Read the model definition and answer for the solid it produces. Units are mm, in the model's axes. A direction names the side the tool comes from. Give positions to 0.01 mm unless a question says otherwise; leave off trailing zeros. Order: outer loops, then holes, each group sorted by start corner. A loop starts at its lowest first (then second) coordinate and runs counter-clockwise, first axis right, second up. Notation, with made-up numbers: (15.5, -2) - (55.5, -2) arc R15 cw to (55.5, 27) - close; hole circle Ø11 at (-39.75, 12). An arc over 180 degrees is marked (long way). Return JSON: item names as keys, results as strings.
Autodesk Inventor part; units mm, degrees
ref_plane "YZ Plane" through (0, 0, 0) normal (1, 0, 0) x (0, 1, 0)
ref_plane "XZ Plane" through (0, 0, 0) normal (0, 1, 0) x (-1, 0, 0)
ref_plane "XY Plane" through (0, 0, 0) normal (0, 0, 1) x (1, 0, 0)
sketch "Sketch1" plane through (0, 0, 0) normal (0, 1, 0) x (-1, 0, 0)
  line L0 (-38.1, 0) -> (38.1, 0)
  line L1 (38.1, 0) -> (38.1, -25.4)
  line L2 (38.1, -25.4) -> (12.7, -25.4)
  line L3 (12.7, -25.4) -> (12.7, -88.9)
  line L4 (12.7, -88.9) -> (-12.7, -88.9)
  line L5 (-12.7, -88.9) -> (-12.7, -25.4)
  line L6 (-12.7, -25.4) -> (-38.1, -25.4)
  line L7 (-38.1, -25.4) -> (-38.1, 0)
  circle A0 centre (0, -12.7) radius 2.4892
  circle A1 centre (25.4, -12.7) radius 2.4892
  line L8 (0, 0) -> (0, -88.9) construction
  circle A2 centre (-25.4, -12.7) radius 2.4892
  circle A3 centre (0, -44.45) radius 2.4892
  circle A4 centre (0, -69.85) radius 2.4892
  point P0 (38.1, -12.7)
  point P1 (0, -44.45)
  dimension "d0" = 76.2
  dimension "d1" = 25.4
  dimension "d2" = 25.4
  dimension "d3" = 63.5
  dimension "d4" = 4.9784
  dimension "d5" = 25.4
  dimension "d6" = 31.75
  dimension "d7" = 25.4
extrude "Extrusion1" add sketch "Sketch1" along normal blind 6.35
fillet "Fillet1" radius 6.35 8 edges at (-38.1, 3.175, 0) (-38.1, 3.175, -25.4) (-12.7, 3.175, -25.4) (-12.7, 3.175, -88.9) (12.7, 3.175, -88.9) (12.7, 3.175, -25.4) (38.1, 3.175, -25.4) (38.1, 3.175, 0)
properties part number "STRU_020_DVBSBracket1" material "Aluminum 6061"
Q1. A cutting plane is placed at C-C (x = 25.4). Write down the section's boundary in (y, z).
Values:
{"outline": "(0, -25.4) - (6.35, -25.4) - (6.35, -15.19) - (0, -15.19) - close; (0, -10.21) - (6.35, -10.21) - (6.35, 0) - (0, 0) - close"}
Q2. Consider L1, parallel to Z at x = 0, y = 2.5; L2, parallel to X at y = 4, z = -13; L3, parallel to X at y = 6, z = -76.5. Determine where each line is inside the solid, lowest interval first.
Values:
{"L1": "z = -88.9 to -72.34, -67.36 to -46.94, -41.96 to -15.19, -10.21 to 0", "L2": "x = -38.1 to -27.87, -22.93 to -2.47, 2.47 to 22.93, 27.87 to 38.1", "L3": "x = -12.7 to 12.7"}
Q3. Given pin 1 (1.5 mm diameter, centred on y = 0.5, z = -65.5, fed in from -X); pin 2 (3 mm diameter, centred on y = 3, z = -69, fed in from +X); pin 3 (3 mm diameter, centred on x = 28, y = 2.5, fed in from -Z), each flat-ended and moving along its own axis, determine where each tip first touches the part or whether it passes through.
Values:
{"pin 1": "stops at x = -12.7", "pin 2": "stops at x = 12.7", "pin 3": "stops at z = -25.4"}
Q4. A cutting plane is placed at B-B (z = -69.85). Write down the section's boundary in (x, y), and give its area (3 significant figures).
Values:
{"outline": "(-12.7, 0) - (-2.49, 0) - (-2.49, 6.35) - (-12.7, 6.35) - close; (2.49, 0) - (12.7, 0) - (12.7, 6.35) - (2.49, 6.35) - close", "area": "130 mm²"}
Q5. For faces 1 (the flat face through (-12.7, 3, -57)), 2 (the flat face through (0, 3, 0)), 3 (the flat face through (25, 3, -25.4)), determine the directions among +Z, -Z, +X, -X, +Y, -Y from which every point of the face is accessible in a straight line to the end or side of a thin tool.
Values:
{"face 1": "-Z, -X, +Y, -Y", "face 2": "+Z, +X, -X, +Y, -Y", "face 3": "-Z, +X, +Y, -Y"}
Q6. Determine the mould class of faces 4 (the flat face through (-25, 3, -25.4)), 5 (the flat face through (12.7, 3, -58)), 6 (the cylindrical face through (-26.74, 3.13, -14.8)) for opening direction Z: released by +Z, released by -Z, zero draft, split by the parting line, or undercut.
Values:
{"face 4": "released by -Z", "face 5": "zero draft", "face 6": "undercut"}
Q7. A cutting plane is placed at A-A (x = 0). Write down the section's boundary in (y, z), and give its area (3 significant figures).
Values:
{"outline": "(0, -88.9) - (6.35, -88.9) - (6.35, -72.34) - (0, -72.34) - close; (0, -67.36) - (6.35, -67.36) - (6.35, -46.94) - (0, -46.94) - close; (0, -41.96) - (6.35, -41.96) - (6.35, -15.19) - (0, -15.19) - close; (0, -10.21) - (6.35, -10.21) - (6.35, 0) - (0, 0) - close", "area": "470 mm²"}
Q8. A cutting plane is placed at D-D (y = 1.75). Write down the section's boundary in (x, z).
Values:
{"outline": "(-38.1, -19.05) arc R6.35 ccw to (-31.75, -25.4) - (-19.05, -25.4) arc R6.35 cw to (-12.7, -31.75) - (-12.7, -82.55) arc R6.35 ccw to (-6.35, -88.9) - (6.35, -88.9) arc R6.35 ccw to (12.7, -82.55) - (12.7, -31.75) arc R6.35 cw to (19.05, -25.4) - (31.75, -25.4) arc R6.35 ccw to (38.1, -19.05) - (38.1, -6.35) arc R6.35 ccw to (31.75, 0) - (-31.75, 0) arc R6.35 ccw to (-38.1, -6.35) - close; hole circle Ø4.98 at (-25.4, -12.7); hole circle Ø4.98 at (0, -69.85); hole circle Ø4.98 at (0, -44.45); hole circle Ø4.98 at (0, -12.7); hole circle Ø4.98 at (25.4, -12.7)"}
